Build history of the part. All positions in model axes, mm. A direction names the side the tool comes from. Round coordinates to 2 decimals unless told otherwise and drop trailing zeros. Write each loop counter-clockwise with the first axis right and the second up, starting at its lowest first coordinate (ties: lowest second). Pieces come first, ordered by that corner, then holes. Notation, with made-up numbers: (54, 86) -> (91, 86) arc R16 ccw to (91, 93) -> close; hole circle Ø6 at (37.5, -28.5). An arc over 180 degrees is marked (long way). Answer as CSV lines item,"result".
from build123d import *

# Parameters (mm, degrees)
SKETCH1_W               = 70
SKETCH1_H               = 35
BOSS_EXTRUDE1_DEPTH     = 2
SKETCH2_W               = 70
SKETCH2_H               = 35
SKETCH2_W_2             = 66
SKETCH2_H_2             = 31
BOSS_EXTRUDE2_DEPTH     = 12
SKETCH3_W               = 56
SKETCH3_H               = 8.5
CUT_EXTRUDE1_DEPTH      = 17
CUT_EXTRUDE1_DEPTH_BACK = 15
SKETCH4_W               = 12
SKETCH4_H               = 2
CUT_EXTRUDE2_DEPTH      = 17
SKETCH5_W               = 9
SKETCH5_H               = 4
SKETCH5_W_2             = 12
SKETCH5_H_2             = 5
CUT_EXTRUDE3_DEPTH      = 17
SKETCH6_W               = 18
SKETCH6_H               = 2
CUT_EXTRUDE4_DEPTH      = 17
SKETCH7_W               = 4
SKETCH7_H               = 1
SKETCH7_W_2             = 20
BOSS_EXTRUDE4_DEPTH     = 1
SKETCH8_W               = 4
SKETCH8_H               = 5
CUT_EXTRUDE5_DEPTH      = 3


with BuildPart() as part:
    # Sketch1 → Boss-Extrude1 (new body)
    with BuildSketch(Plane(origin=(0, 0, 0), x_dir=(1, 0, 0), z_dir=(0, 1, 0))):
        with Locations((35, 17.5)):
            Rectangle(SKETCH1_W, SKETCH1_H)
    extrude(amount=BOSS_EXTRUDE1_DEPTH)

    # Sketch2 → Boss-Extrude2 (add)
    with BuildSketch(Plane(origin=(0, 2, 0), x_dir=(1, 0, 0), z_dir=(0, 1, 0))):
        with Locations((35, 17.5)):
            Rectangle(SKETCH2_W, SKETCH2_H)
        with Locations((35, 17.5)):
            Rectangle(SKETCH2_W_2, SKETCH2_H_2, mode=Mode.SUBTRACT)
    extrude(amount=BOSS_EXTRUDE2_DEPTH)

    # Sketch3 → Cut-Extrude1 (cut, two sides)
    with BuildSketch(Plane(origin=(0, 2, 0), x_dir=(1, 0, 0), z_dir=(0, 1, 0))) as cut_extrude1_sk:
        with Locations((35, 30.75)):
            Rectangle(SKETCH3_W, SKETCH3_H)
    extrude(amount=CUT_EXTRUDE1_DEPTH, mode=Mode.SUBTRACT)
    extrude(cut_extrude1_sk.sketch, amount=-CUT_EXTRUDE1_DEPTH_BACK, mode=Mode.SUBTRACT)

    # Sketch4 → Cut-Extrude2 (cut)
    with BuildSketch(Plane.ZY.offset(-68)):
        with Locations((-21, 13)):
            Rectangle(SKETCH4_W, SKETCH4_H)
    extrude(amount=-CUT_EXTRUDE2_DEPTH, mode=Mode.SUBTRACT)

    # Sketch5 → Cut-Extrude3 (cut)
    with BuildSketch(Plane(origin=(0, 0, -2), x_dir=(-1, 0, 0), z_dir=(0, 0, -1))):
        with Locations((-12.5, 12)):
            Rectangle(SKETCH5_W, SKETCH5_H)
        with Locations((-25.5, 12)):
            Rectangle(SKETCH5_W, SKETCH5_H)
        with Locations((-56, 11.5)):
            Rectangle(SKETCH5_W_2, SKETCH5_H_2)
    extrude(amount=-CUT_EXTRUDE3_DEPTH, mode=Mode.SUBTRACT)

    # Sketch6 → Cut-Extrude4 (cut)
    with BuildSketch(Plane(origin=(2, 0, 0), x_dir=(0, 0, -1), z_dir=(1, 0, 0))):
        with Locations((19, 13)):
            Rectangle(SKETCH6_W, SKETCH6_H)
    extrude(amount=-CUT_EXTRUDE4_DEPTH, mode=Mode.SUBTRACT)

    # Sketch7 → Boss-Extrude4 (add)
    with BuildSketch(Plane(origin=(0, 14, 0), x_dir=(1, 0, 0), z_dir=(0, 1, 0))):
        Polygon((7, 33), (7, 34), (1, 34), (1, 28), (2, 28), (2, 33), align=None)
        Polygon((2, 10), (1, 10), (1, 1), (8, 1), (8, 2), (2, 2), align=None)
        with Locations((19, 1.5)):
            Rectangle(SKETCH7_W, SKETCH7_H)
        with Locations((40, 1.5)):
            Rectangle(SKETCH7_W_2, SKETCH7_H)
        Polygon((69, 1), (69, 15), (68, 15), (68, 2), (62, 2), (62, 1), align=None)
        Polygon((68, 27), (69, 27), (69, 34), (63, 34), (63, 33), (68, 33), align=None)
    extrude(amount=BOSS_EXTRUDE4_DEPTH)

    # Sketch8 → Cut-Extrude5 (cut)
    with BuildSketch(Plane(origin=(0, 0, -2), x_dir=(-1, 0, 0), z_dir=(0, 0, -1))):
        with Locations((-19, 12.5)):
            Rectangle(SKETCH8_W, SKETCH8_H)
    extrude(amount=-CUT_EXTRUDE5_DEPTH, mode=Mode.SUBTRACT)


solid = part.part
1. Probe line 1 along X through (y, z) = (7.25, -7); line 2 along X through (y, z) = (1.75, -32.5); line 3 along Z through (x, y) = (65.5, 4.5). List the from-to ranges inside material, lowest first.
Results found:
line 1,"x = 0 to 2, 68 to 70"
line 2,"x = 0 to 7, 63 to 70"
line 3,"z = -35 to -33, -2 to 0"
2. Mould opens along Z. For faces 6 (the flat face through (1, 13, -10)), 7 (the flat face through (66, 7, -35)), 8 (the flat face through (69.3, 14, -32.5)), 9 (the flat face through (1, 13, -28)) say: +Z half, -Z half, draft (parallel to the pull), parting line (faces both ways), or undercut.
Results found:
face 6,"undercut"
face 7,"-Z half"
face 8,"draft"
face 9,"undercut"
3. Cut at D-D, the plane z = -8.5. Write the cut outline in (x, y), then the cut area to 3 significant figures.
Results found:
outline,"(0, 0) -> (70, 0) -> (70, 14) -> (69, 14) -> (69, 15) -> (68, 15) -> (68, 2) -> (2, 2) -> (2, 15) -> (1, 15) -> (1, 14) -> (0, 14) -> close"
area,"190 mm2"
4. Cut at C-C, the plane y = 7.75. Write the cut outline in (x, z).
Results found:
outline,"(0, -35) -> (7, -35) -> (7, -33) -> (2, -33) -> (2, -2) -> (68, -2) -> (68, -33) -> (63, -33) -> (63, -35) -> (70, -35) -> (70, 0) -> (0, 0) -> close"
5. Cut at A-A, the plane z = -32. Write the cut outline in (x, y), then the cut area to 3 significant figures.
Results found:
outline,"(0, 0) -> (7, 0) -> (7, 2) -> (2, 2) -> (2, 15) -> (1, 15) -> (1, 14) -> (0, 14) -> close; (63, 0) -> (70, 0) -> (70, 14) -> (69, 14) -> (69, 15) -> (68, 15) -> (68, 2) -> (63, 2) -> close"
area,"78.0 mm2"
6. Which spindle directions (+Z, -Z, +X, -X, +Y, -Y) get a long thin tool onto all of the face, cutting with end or side? Do faces 1 (the flat face through (30, 12, -1)), 2 (the flat face through (1.6, 15, -4.2)), 3 (the flat face through (35, 1, -26.5)), 4 (the flat face through (4, 8, -33)), 5 (the flat face through (1, 12, -19)). Say none if no direction does.
Results found:
face 1,"+Z, -Z, +Y"
face 2,"+Z, -Z, +X, -X, +Y"
face 3,"-Z, +Y, -Y"
face 4,"+Y"
face 5,"-X, +Y"
7. Drop flat-ended pins along their axis: pin 1 Ø0.6 at (y, z) = (12.5, -1) entering from -X; pin 2 Ø1.5 at (x, z) = (50.5, -28) entering from +Y (3 decimals); pin 3 Ø2 at (x, z) = (1, -21.5) entering from +Y; pin 4 Ø4 at (x, y) = (30, 10) entering from -Z. Give the stop position or say it passes through.
Results found:
pin 1,"stops at x = 0"
pin 2,"passes through"
pin 3,"stops at y = 12"
pin 4,"stops at z = -2"
8. Cut at B-B, the plane y = 11. Write the cut outline in (x, z).
Results found:
outline,"(0, -35) -> (7, -35) -> (7, -33) -> (2, -33) -> (2, -2) -> (8, -2) -> (8, 0) -> (0, 0) -> close; (30, -2) -> (50, -2) -> (50, 0) -> (30, 0) -> close; (62, -2) -> (68, -2) -> (68, -33) -> (63, -33) -> (63, -35) -> (70, -35) -> (70, 0) -> (62, 0) -> close"
